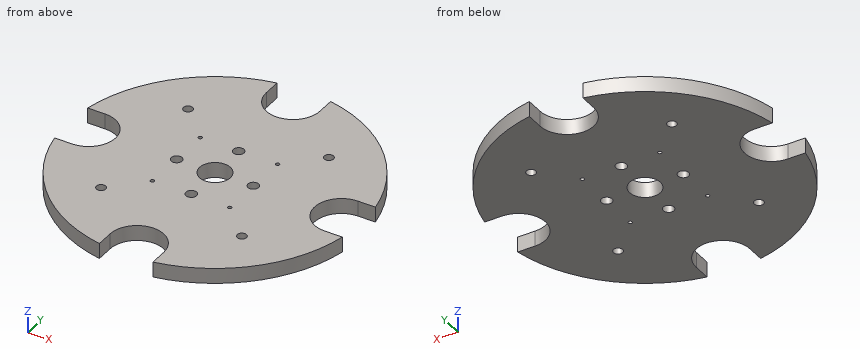
from build123d import *

# Parameters (mm, degrees)
ESQUISSE1_R                  = 191
BASE_EXTRUSION_DEPTH         = 20
ESQUISSE2_R                  = 20
ENL_V_MAT_EXTRU_1_DEPTH      = 20
ESQUISSE3_R                  = 7
ENL_V_MAT_EXTRU_2_DEPTH      = 20
R_P_TITION_CIRCULAIRE1_COUNT = 4
ESQUISSE4_R                  = 6
ESQUISSE4_R_2                = 2.5
ENL_V_MAT_EXTRU_3_DEPTH      = 20
R_P_TITION_CIRCULAIRE2_COUNT = 4
ENL_V_MAT_EXTRU_4_DEPTH      = 271.854204324
R_P_TITION_CIRCULAIRE3_COUNT = 4


with BuildPart() as part:
    # Esquisse1 → Base-Extrusion (new body)
    with BuildSketch(Plane.XY):
        Circle(ESQUISSE1_R)
    extrude(amount=BASE_EXTRUSION_DEPTH)

    # Esquisse2 → Enlèv. mat.-Extru.1 (cut)
    with BuildSketch(Plane.XY.offset(20)):
        Circle(ESQUISSE2_R)
    extrude(amount=-ENL_V_MAT_EXTRU_1_DEPTH, mode=Mode.SUBTRACT)

    # Esquisse3 → Enlèv. mat.-Extru.2 (cut)
    with BuildSketch(Plane.XY.offset(20)):
        with Locations((50, 0)):
            Circle(ESQUISSE3_R)
    enl_v_mat_extru_2 = extrude(amount=-ENL_V_MAT_EXTRU_2_DEPTH, mode=Mode.SUBTRACT)

    # Répétition circulaire1: Enlèv. mat.-Extru.2 ×4 about axis
    r_p_tition_circulaire1_axis = Axis((0, 0, 0), (0, 0, -1))
    for i in range(1, R_P_TITION_CIRCULAIRE1_COUNT):
        add(enl_v_mat_extru_2.rotate(r_p_tition_circulaire1_axis, i * 360 / R_P_TITION_CIRCULAIRE1_COUNT), mode=Mode.SUBTRACT)

    # Esquisse4 → Enlèv. mat.-Extru.3 (cut)
    with BuildSketch(Plane.XY.offset(20)):
        with Locations((91.923881554, 91.923881554)):
            Circle(ESQUISSE4_R)
        with Locations((50.558134855, 50.558134855)):
            Circle(ESQUISSE4_R_2)
    enl_v_mat_extru_3 = extrude(amount=-ENL_V_MAT_EXTRU_3_DEPTH, mode=Mode.SUBTRACT)

    # Répétition circulaire2: Enlèv. mat.-Extru.3 ×4 about axis
    r_p_tition_circulaire2_axis = Axis((0, 0, 0), (0, 0, -1))
    for i in range(1, R_P_TITION_CIRCULAIRE2_COUNT):
        add(enl_v_mat_extru_3.rotate(r_p_tition_circulaire2_axis, i * 360 / R_P_TITION_CIRCULAIRE2_COUNT), mode=Mode.SUBTRACT)

    # Esquisse5 → Enlèv. mat.-Extru.4 (cut, through all)
    with BuildSketch(Plane.XY.offset(20)):
        with BuildLine():
            Line((-35, 187.765811585), (-35, 165))
            ThreePointArc((-35, 165), (0, 130), (35, 165))
            Line((35, 165), (35, 187.765811585))
            ThreePointArc((35, 187.765811585), (0, 191), (-35, 187.765811585))
        make_face()
    enl_v_mat_extru_4 = extrude(amount=-ENL_V_MAT_EXTRU_4_DEPTH, mode=Mode.SUBTRACT)

    # Répétition circulaire3: Enlèv. mat.-Extru.4 ×4 about axis
    r_p_tition_circulaire3_axis = Axis((0, 0, 0), (0, 0, -1))
    for i in range(1, R_P_TITION_CIRCULAIRE3_COUNT):
        add(enl_v_mat_extru_4.rotate(r_p_tition_circulaire3_axis, i * 360 / R_P_TITION_CIRCULAIRE3_COUNT), mode=Mode.SUBTRACT)


solid = part.part
Source: CAD feature listing. Evaluate the final solid. Frame: model axes, mm. Coordinates: 2 decimals unless noted, no trailing zeros. Loops run counter-clockwise (first coordinate to the right, second up) from the corner with the lowest first, then second, coordinate; pieces in that order, holes last. Notation, with made-up numbers: (58, 21.25) - (100, 21.25) arc R30 cw to (100, 48.25) - close; hole circle Ø9 at (-23, -35). An arc over 180 degrees is marked (long way). One line per item, written item: value. Start each with the question number.
1. Ray query, L1, parallel to Y at x = -50, z = 7.5; L2, parallel to Y at x = -95, z = 6.5. Return the intervals inside material, ascending.
2. Section C-C (z = 12.5). State how many separate pieces and enclosed holes the cut face has, and give its area (3 significant figures).
3. Contact query for flat-ended pins moving along their axis: P1, Ø22.5, axis at x = -50, y = 0, coming from the -Z side; P2, Ø12, axis at x = -0.5, z = 5.5, coming from the +Y side; P3, Ø4, axis at x = -50.56, y = -50.56, coming from the -Z side; P4, Ø10, axis at y = -175.5, z = 9, coming from the +X side. Output: stop coordinate, or through.
4. Section B-B (x = 136). Return the cut outline in (y, z), and give its area (3 significant figures).
5. Section D-D (x = -136.5). Return the cut outline in (y, z), and give its area (3 significant figures).
6. Section A-A (y = 0). Return the cut outline in (x, z).
Verdict:
1. L1: y = -184.34 to -53, -48.12 to -7, 7 to 48.12, 53 to 184.34
1. L2: y = -165.7 to -97.08, -86.77 to 86.77, 97.08 to 165.7
2. separate pieces: 1
2. enclosed holes: 13
2. area: 97,500 mm2
3. P1: stops at z = 0
3. P2: stops at y = 130.61
3. P3: passes through
3. P4: stops at x = 86.09
4. outline: (-134.11, 0) - (-19.6, 0) - (-19.6, 20) - (-134.11, 20) - close; (19.6, 0) - (134.11, 0) - (134.11, 20) - (19.6, 20) - close
4. area: 4,580 mm2
5. outline: (-133.6, 0) - (-20.32, 0) - (-20.32, 20) - (-133.6, 20) - close; (20.32, 0) - (133.6, 0) - (133.6, 20) - (20.32, 20) - close
5. area: 4,530 mm2
6. outline: (-130, 0) - (-57, 0) - (-57, 20) - (-130, 20) - close; (-43, 0) - (-20, 0) - (-20, 20) - (-43, 20) - close; (20, 0) - (43, 0) - (43, 20) - (20, 20) - close; (57, 0) - (130, 0) - (130, 20) - (57, 20) - close
